Geometry: final body of the model. Coordinates: model frame, mm. Give positions to 0.01 mm unless a question says otherwise; leave off trailing zeros. Write item = value, one per line. Start each with the question number.
from build123d import *

# Parameters (mm, degrees)
BOSS_EXTRU_1_DEPTH           = 1
ENL_V_MAT_EXTRU_1_DEPTH      = 144.780695976
ENL_V_MAT_EXTRU_1_DEPTH_BACK = 144.780695976
ESQUISSE2_R                  = 1.6


with BuildPart() as part:
    # Esquisse1 → Boss.-Extru.1 (new body)
    with BuildSketch(Plane.XY):
        with BuildLine():
            Line((26.971910928, 14.707354998), (78.971910928, 14.707354998))
            ThreePointArc((78.971910928, 14.707354998), (82.507444834, 16.171821092), (83.971910928, 19.707354998))
            Line((83.971910928, 19.707354998), (83.971910928, 111.707354998))
            ThreePointArc((83.971910928, 111.707354998), (82.507444834, 115.242888904), (78.971910928, 116.707354998))
            Line((78.971910928, 116.707354998), (26.971910928, 116.707354998))
            ThreePointArc((26.971910928, 116.707354998), (23.436377022, 115.242888904), (21.971910928, 111.707354998))
            Line((21.971910928, 111.707354998), (21.971910928, 19.707354998))
            ThreePointArc((21.971910928, 19.707354998), (23.436377022, 16.171821092), (26.971910928, 14.707354998))
        make_face()
    extrude(amount=BOSS_EXTRU_1_DEPTH)

    # Esquisse2 → Enlèv. mat.-Extru.1 (cut, two sides: drawn at the far end of the back side and taken through both)
    with BuildSketch(Plane.XY.offset(1).offset(-ENL_V_MAT_EXTRU_1_DEPTH_BACK)):
        with Locations((27.143483803, 19.878927873)):
            Circle(ESQUISSE2_R)
        with Locations((78.800338052, 19.878927873)):
            Circle(ESQUISSE2_R)
        with Locations((27.143483803, 111.535782123)):
            Circle(ESQUISSE2_R)
        with Locations((78.800338052, 111.535782123)):
            Circle(ESQUISSE2_R)
    extrude(amount=ENL_V_MAT_EXTRU_1_DEPTH + ENL_V_MAT_EXTRU_1_DEPTH_BACK, mode=Mode.SUBTRACT)


solid = part.part
Q1. Material intervals for line 1 along X through (y, z) = (21, 0.1); line 2 along Y through (x, z) = (77.5, 0.2); line 3 along Y through (x, z) = (25, 0.15), sorted ascending. Write a range as from..to.
Q2. Pull-direction query (X, two-part tool) for faces 1 (the flat face through (53, 66, 0)), 2 (the cylindrical face through (25.545, 19.949, 0.493)), 3 (the cylindrical face through (82.468, 16.133, 0.493)), 4 (the cylindrical face through (79.539, 110.116, 0.493)); classes: +X half, -X half, draft (parallel to the pull), parting line (faces both ways), or undercut.
Q3. Contact query for a flat-ended pin moving along its axis: pin 1 (3.5 mm diameter, centred on x = 27.14, y = 111.54, fed in from +Z). Output: stop coordinate, or through.
The answers:
q1.line_1 = 21.97..26, 28.29..77.66, 79.94..83.97
q1.line_2 = 14.71..18.95, 20.81..110.6, 112.47..116.71
q1.line_3 = 15.11..116.3
q2.face_1 = draft
q2.face_2 = undercut
q2.face_3 = +X half
q2.face_4 = undercut
q3.pin_1 = 1
